The listing builds one solid part. Answer for the finished solid, in the listing's coordinates (mm). Face numbers are marked on the shaded views. A direction names the side the tool comes from. Coordinates: 2 decimals unless noted, no trailing zeros. Write each loop counter-clockwise with the first axis right and the second up, starting at its lowest first coordinate (ties: lowest second). Pieces come first, ordered by that corner, then holes. Notation, with made-up numbers: M 68,-1 L 108,-1 A10 cw 108,12 Z; hole C 0.25,-16 d8. An arc over 180 degrees is marked long. Answer as a JSON object with one key per item and string values. Group by question number.
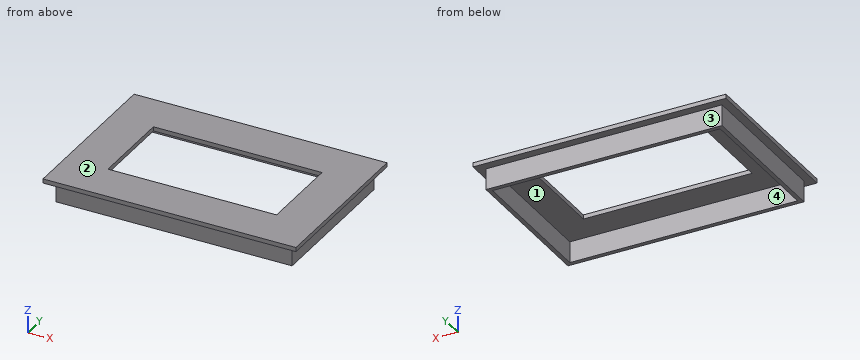
from build123d import *

# Parameters (mm, degrees)
SKETCH1_W           = 56
SKETCH1_H           = 36
SKETCH1_W_2         = 54
SKETCH1_H_2         = 34
BOSS_EXTRUDE1_DEPTH = 5
SKETCH3_W           = 60
SKETCH3_H           = 40
BOSS_EXTRUDE3_DEPTH = 1
SKETCH4_W           = 40
SKETCH4_H           = 20
CUT_EXTRUDE2_DEPTH  = 7


with BuildPart() as part:
    # Sketch1 → Boss-Extrude1 (new body)
    with BuildSketch(Plane.XY):
        Rectangle(SKETCH1_W, SKETCH1_H)
        Rectangle(SKETCH1_W_2, SKETCH1_H_2, mode=Mode.SUBTRACT)
    extrude(amount=BOSS_EXTRUDE1_DEPTH)

    # Sketch3 → Boss-Extrude3 (add)
    with BuildSketch(Plane.XY.offset(5)):
        Rectangle(SKETCH3_W, SKETCH3_H)
    extrude(amount=BOSS_EXTRUDE3_DEPTH)

    # Sketch4 → Cut-Extrude2 (cut, through all)
    with BuildSketch(Plane.XY.offset(6)):
        Rectangle(SKETCH4_W, SKETCH4_H)
    extrude(amount=-CUT_EXTRUDE2_DEPTH, mode=Mode.SUBTRACT)


solid = part.part
Item 1: Consider L1, parallel to Y at x = 22, z = 1.05; L2, parallel to X at y = -13, z = 2.15; L3, parallel to X at y = -3.5, z = 5.15. Determine where each line is inside the solid, lowest interval first. Write a range as from..to.
Item 2: A cutting plane is placed at D-D, the plane x = -22.5. Write down the section's boundary in (y, z).
Item 3: A cutting plane is placed at B-B, the plane y = -4. Write down the section's boundary in (x, z).
Item 4: For a pull along X with two mould halves and no side action, classify the marked faces 1 and 2 as +X half, -X half, draft (parallel to the pull), parting line (faces both ways), or undercut.
Item 5: A tool of negligible diameter and unlimited length cuts with its end or side. For the marked faces 3 and 4, from which of +Z, -Z, +X, -X, +Y, -Y can it reach the whole face along a straight path? Write none if from no direction.
Item 6: Flat-ended cylindrical pins translate along their axes: pin 1 Ø20 at (x, y) = (10.5, -4.5) entering from -Z; pin 2 Ø2.5 at (x, z) = (6.5, 2) entering from +Y; pin 3 Ø1.5 at (y, z) = (7.5, 3) entering from -X. Find the tip coordinate at first contact, or state that the pin passes through.
Item 7: A cutting plane is placed at C-C, the plane x = -14.5. Write down the section's boundary in (y, z).
Item 8: A cutting plane is placed at A-A, the plane z = 0.9. Write down the section's boundary in (x, y).
Answer:
{
 "1": {"L1": "-18..-17, 17..18", "L2": "-28..-27, 27..28", "L3": "-30..-20, 20..30"},
 "2": {"outline": "M -20,5 L -18,5 L -18,0 L -17,0 L -17,5 L 17,5 L 17,0 L 18,0 L 18,5 L 20,5 L 20,6 L -20,6 Z"},
 "3": {"outline": "M -30,5 L -28,5 L -28,0 L -27,0 L -27,5 L -20,5 L -20,6 L -30,6 Z; M 20,5 L 27,5 L 27,0 L 28,0 L 28,5 L 30,5 L 30,6 L 20,6 Z"},
 "4": {"face 1": "undercut", "face 2": "draft"},
 "5": {"face 3": "-Z, +X, -X, +Y", "face 4": "-Z"},
 "6": {"pin 1": "z = 5", "pin 2": "y = 18", "pin 3": "x = -28"},
 "7": {"outline": "M -20,5 L -18,5 L -18,0 L -17,0 L -17,5 L -10,5 L -10,6 L -20,6 Z; M 10,5 L 17,5 L 17,0 L 18,0 L 18,5 L 20,5 L 20,6 L 10,6 Z"},
 "8": {"outline": "M -28,-18 L 28,-18 L 28,18 L -28,18 Z; hole M -27,-17 L 27,-17 L 27,17 L -27,17 Z"}
}
